Autodesk Inventor part; units mm, degrees
ref_plane "YZ Plane" through (0, 0, 0) normal (1, 0, 0) x (0, 1, 0)
ref_plane "XZ Plane" through (0, 0, 0) normal (0, 1, 0) x (-1, 0, 0)
ref_plane "XY Plane" through (0, 0, 0) normal (0, 0, 1) x (1, 0, 0)
sketch "Sketch1" plane through (0, 0, 0) normal (0, 0, 1) x (1, 0, 0)
  line L0 (-33.8571, 0) -> (-33.8571, 3)
  line L1 (-33.8571, 3) -> (-56.4286, 3)
  line L2 (-56.4286, 3) -> (-56.4286, 0)
  line L3 (11.2857, 0) -> (11.2857, 3)
  line L4 (11.2857, 3) -> (-11.2857, 3)
  line L5 (-11.2857, 3) -> (-11.2857, 0)
  line L6 (56.4286, 0) -> (56.4286, 3)
  line L7 (56.4286, 3) -> (33.8571, 3)
  line L8 (33.8571, 3) -> (33.8571, 0)
  line L9 (-79, 22) -> (-79, 22)
  line L10 (-79, 22) -> (-79, 11)
  line L11 (-79, 11) -> (-79, 11)
  line L12 (79, 11) -> (79, 11)
  line L13 (79, 11) -> (79, 22)
  line L14 (79, 22) -> (79, 22)
  line L15 (-56.4286, 33) -> (-79, 33)
  line L16 (79, 33) -> (56.4286, 33)
  line L17 (33.8571, 33) -> (11.2857, 33)
  line L18 (-11.2857, 33) -> (-33.8571, 33)
  line L19 (79, 0) -> (79, 11)
  line L20 (79, 22) -> (79, 33)
  line L21 (56.4286, 0) -> (79, 0)
  line L22 (11.2857, 0) -> (33.8571, 0)
  line L23 (-79, 0) -> (-56.4286, 0)
  line L24 (-33.8571, 0) -> (-11.2857, 0)
  line L25 (-79, 33) -> (-79, 22)
  line L26 (-79, 11) -> (-79, 0)
  line L27 (-56.4286, 33) -> (57.8569, 33)
  point P0 (0, 0)
  point P1 (0, 30)
  point P2 (52.5, 33)
  dimension "d46" = 158
  dimension "d48" = 33
  dimension "d49" = 79
  dimension "d50" = 0
  dimension "d53" = 0
  dimension "d58" = 11
  dimension "d59" = 11
  dimension "d61" = 22.5714
  dimension "d62" = 11.2857
  dimension "d63" = 0
  dimension "d64" = 0
  dimension "d65" = 3
extrude "Extrusion1" add sketch "Sketch1" along normal blind 3
sketch "Sketch3" plane through (0, 0, 3) normal (0, 0, 1) x (1, 0, 0)
  line L0 (-79, 33) -> (-79, 0)
  line L1 (-79, 33) -> (-76, 33)
  line L2 (-76, 33) -> (-76, 22)
  line L3 (-76, 22) -> (-79, 22)
  line L4 (-79, 22) -> (-79, 33)
  line L5 (-79, 0) -> (-56.4286, 0)
  line L6 (-79, 0) -> (-76, 0)
  line L7 (-76, 0) -> (-76, 11)
  line L8 (-76, 11) -> (-79, 11)
  line L9 (-79, 11) -> (-79, 0)
  line L10 (79, 33) -> (-79, 33)
  line L11 (79, 33) -> (76, 33)
  line L12 (76, 33) -> (76, 22)
  line L13 (76, 22) -> (79, 22)
  line L14 (79, 22) -> (79, 33)
  line L15 (79, 0) -> (79, 33)
  line L16 (79, 0) -> (76, 0)
  line L17 (76, 0) -> (76, 11)
  line L18 (76, 11) -> (79, 11)
  line L19 (79, 11) -> (79, 0)
  point P0 (0, 0)
  dimension "d66" = 11
  dimension "d67" = 3
extrude "Extrusion3" cut sketch "Sketch3" against normal through all
equation "\"d46\" = shelfWs"
equation "\"d48\" = shelfD"
equation "\"d58\" = 0.333333 * shelfD - tol"
equation "\"d59\" = 0.333333 * shelfD + 2 * tol"
equation "\"d24\" = tt"
equation "\"d0\" = 0.5 * shelfWs"
equation "\"tt\" = 3"
equation "\"tol\" = 0"
equation "\"d2\" = shelfD"
equation "\"d4\" = tt"
equation "\"tiroir\" = 1"
equation "\"nHoles\" = 4"
equation "\"shelfH\" = 35"
equation "\"shelfWs\" = 158"
equation "\"d47\" = 0.5 * shelfWs"
properties part number "back"
Could you check a few things on this model? Use its own coordinates, in mm. A direction names the side the tool comes from. Round coordinates to 2 decimals unless told otherwise and drop trailing zeros. Write each loop counter-clockwise with the first axis right and the second up, starting at its lowest first coordinate (ties: lowest second). Pieces come first, ordered by that corner, then holes. Notation, with made-up numbers: M 76.25,-12 L 96.25,-12 A25 ccw 96.25,7 Z; hole C 73,35.5 d3. An arc over 180 degrees is marked long. Answer in a Markdown table with one row per item. Add a question column.
Q1. Imagine slicing it at C-C (y = 4.5). Please give me the cut outline in (x, z).
Q2. Imagine slicing it at B-B (x = 49). Please give me the cut outline in (y, z).
Q3. Will these pins go through, and if not, where does the flat tip stop? pin 1 Ø0.9 at (y, z) = (28.5, 1.5) entering from +X; pin 2 Ø1.5 at (x, z) = (-26.5, 1.5) entering from -Y; pin 3 Ø0.9 at (x, z) = (45.5, 2) entering from -Y; pin 4 Ø1.5 at (y, z) = (2, 1.5) entering from -X.
Q4. On a 3-axis mill with a long thin cutter (end or side, diameter ignored), from which of +Z, -Z, +X, -X, +Y, -Y can I reach the whole of each face in a straight line? I mean faces 4 (the flat face through (77, 11, 2)), 5 (the flat face through (-77, 22, 2)), 6 (the flat face through (33.857, 2, 1)). Say none if no direction works.
Q5. If we mould it in two halves opening along X, with no side actions, what happens to faces 1 (the flat face through (-79, 17, 1)), 2 (the flat face through (22, 0, 1)), 3 (the flat face through (-56.429, 2, 1))? For each: +X half, -X half, draft (parallel to the pull), parting line (faces both ways), or undercut.
Q6. If I drill on line 1 (Y direction, x = 49, z = 0.95); line 2 (X direction, y = 27, z = 2.6), over which ranges is the centre line in solid material (lowest first)? Write a range as from..to.
Q7. Imagine slicing it at A-A (z = 1.05). Please give me the cut outline in (x, y), then the cut area to 3 significant figures.
Values:
| question | item | result |
|---|---|---|
| 1 | outline | M -76,0 L 76,0 L 76,3 L -76,3 Z |
| 2 | outline | M 3,0 L 33,0 L 33,3 L 3,3 Z |
| 3 | pin 1 | x = 76 |
| 3 | pin 2 | y = 0 |
| 3 | pin 3 | y = 3 |
| 3 | pin 4 | x = -76 |
| 4 | face 4 | +Z, -Z, +X, -Y |
| 4 | face 5 | +Z, -Z, -X, +Y |
| 4 | face 6 | +Z, -Z, -Y |
| 5 | face 1 | -X half |
| 5 | face 2 | draft |
| 5 | face 3 | undercut |
| 6 | line 1 | 3..33 |
| 6 | line 2 | -76..76 |
| 7 | outline | M -79,11 L -76,11 L -76,0 L -56.43,0 L -56.43,3 L -33.86,3 L -33.86,0 L -11.29,0 L -11.29,3 L 11.29,3 L 11.29,0 L 33.86,0 L 33.86,3 L 56.43,3 L 56.43,0 L 76,0 L 76,11 L 79,11 L 79,22 L 76,22 L 76,33 L -76,33 L -76,22 L -79,22 Z |
| 7 | area | 4,880 mm^2 |
